Job drawing, mm, ordinate dimensions from the low corner. One solid piece. A direction names the side the tool comes from. Round coordinates to 2 decimals unless told otherwise and drop trailing zeros. Write each loop counter-clockwise with the first axis right and the second up, starting at its lowest first coordinate (ties: lowest second). Pieces come first, ordered by that corner, then holes. Notation, with made-up numbers: (30, -38) -> (43, -38) arc R14 ccw to (43, -21) -> close; hole circle Ø6 at (-11, 48). An arc over 180 degrees is marked (long way). Use CSV: the item, a comma, the result in double quotes. Start each with the question number.
(1) Saw through at D-D (x = 31.5). Give the cut face in (y, z).
(2) Probe line 1 (Y direction, x = 15, z = 28.5); line 2 (Z direction, x = 14.5, y = 1.55); line 3 (Z direction, x = 18, y = 0.75). List the from-to ranges inside material, lowest first. Write a range as [from, to].
(3) Saw through at C-C (y = 1.85). Give the cut face in (x, z), plus the area to 3 significant figures.
(4) Saw through at A-A (z = 17.5). Give the cut face in (x, y).
(5) Drop flat-ended pins along their axis: pin 1 (4 mm diameter, centred on x = 5.5, z = 13, fed in from -Y); pin 2 (6 mm diameter, centred on x = 3.5, z = 10.5, fed in from +Y). Give the stop position or say it passes through.
(6) Two-plate mould, pull along Z, no slides. Class the marked faces 1 and 2: released by +Z, released by -Z, zero draft, split by the parting line, or undercut.
(7) Which spindle directions (+Z, -Z, +X, -X, +Y, -Y) get a long thin tool onto all of the face, cutting with end or side? Do the marked faces 3, 4 and 5. Say none if no direction does.
(8) Saw through at B-B (x = 17.5). Give the cut face in (y, z), plus the area to 3 significant figures.
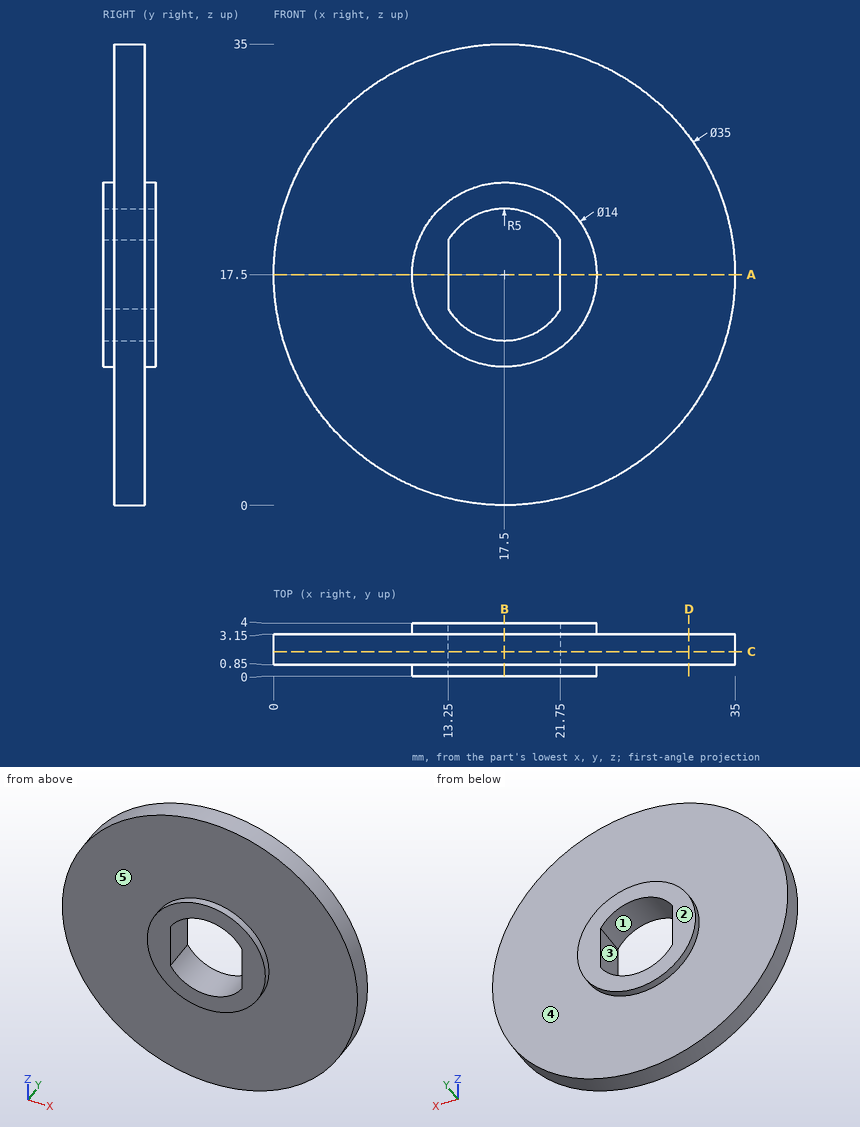
Answers:
1,outline,"(0.85, 7) -> (3.15, 7) -> (3.15, 28) -> (0.85, 28) -> close"
2,line 1,"y = [0.85, 3.15]"
2,line 2,"z = [0.26, 13.5], [21.5, 34.74]"
2,line 3,"z = [10.52, 12.53], [22.47, 24.48]"
3,outline,"circle Ø35 at (17.5, 17.5); hole (13.25, 14.87) arc R5 ccw to (21.75, 14.87) -> (21.75, 20.13) arc R5 ccw to (13.25, 20.13) -> close"
3,area,"889 mm²"
4,outline,"(0, 0.85) -> (10.5, 0.85) -> (10.5, 0) -> (13.25, 0) -> (13.25, 4) -> (10.5, 4) -> (10.5, 3.15) -> (0, 3.15) -> close; (21.75, 0) -> (24.5, 0) -> (24.5, 0.85) -> (35, 0.85) -> (35, 3.15) -> (24.5, 3.15) -> (24.5, 4) -> (21.75, 4) -> close"
5,pin 1,"stops at y = 0.85"
5,pin 2,"stops at y = 3.15"
6,face 1,"undercut"
6,face 2,"zero draft"
7,face 3,"+Y, -Y"
7,face 4,"+Y"
7,face 5,"-Y"
8,outline,"(0, 10.5) -> (0.85, 10.5) -> (0.85, 0) -> (3.15, 0) -> (3.15, 10.5) -> (4, 10.5) -> (4, 12.5) -> (0, 12.5) -> close; (0, 22.5) -> (4, 22.5) -> (4, 24.5) -> (3.15, 24.5) -> (3.15, 35) -> (0.85, 35) -> (0.85, 24.5) -> (0, 24.5) -> close"
8,area,"64.3 mm²"
